The listing builds one solid part. Answer for the finished solid, in the listing's coordinates (mm). A direction names the side the tool comes from. Coordinates: 2 decimals unless noted, no trailing zeros. Loops run counter-clockwise (first coordinate to the right, second up) from the corner with the lowest first, then second, coordinate; pieces in that order, holes last. Notation, with made-up numbers: M 43,57.25 L 68,57.25 A23 ccw 68,83.25 Z; hole C 46.25,44.25 d4. An arc over 180 degrees is marked long. Return JSON: item names as keys, results as strings. Group by question number.
1. Section D-D (z = 17.5) is taken. Write down the section's boundary in (x, y).
2. Section C-C (z = -3.5) is taken. Write down the section's boundary in (x, y).
3. Which of the six approach directions +Z, -Z, +X, -X, +Y, -Y give full straight-line access (tool end or side, diameter ignored) to faces 5 (the face through (-24.6, 2, 0)), 6 (the face through (1.14, 1.48, -59.99))?
4. Section B-B (y = 1.5) is taken. Count the separate pieces of the cut face and the enclosed holes in it, then the cut area to 3 significant figures.
5. The mould has two halves that part along Z. Classify faces 1 (the face through (-1, 3, -1)), 2 (the face through (-41, 2, -12.9)), 3 (the face through (42, 2, -12.9)), 4 (the face through (-1.14, 1.48, 59.99)): pulls with the +Z half, pulls with the -Z half, needs draft (parallel to the pull), parting line crosses it, or undercut.
6. Given P1, Ø2, axis at x = -24.07, z = -45.64, coming from the -Y side; P2, Ø3, axis at x = -19, z = -14.5, coming from the -Y side; P3, Ø1.5, axis at y = 1.5, z = 0, coming from the -X side; P4, Ø1.4, axis at x = -27.5, y = 1, coming from the -Z side, each flat-ended and moving along its own axis, determine where each tip first touches the part or whether it passes through.
7. Section A-A (x = -30) is taken. Write down the section's boundary in (y, z).
8. Straight lines are drawn through the part: L1, parallel to Z at x = -25, y = 2.85; L2, parallel to Z at x = -39, y = 1.55; L3, parallel to Z at x = -0.5, y = 1.1. For each, find the intervals that lie inside material, in ascending order. Write a range as from..to.
```python
from build123d import *

# Parameters (mm, degrees)
SKETCH1_R           = 60
BOSS_EXTRUDE1_DEPTH = 3
SKETCH2_R           = 1.25
CUT_EXTRUDE1_DEPTH  = 4
CUT_EXTRUDE9_DEPTH  = 4
SKETCH5_R           = 0.9
BOSS_EXTRUDE2_DEPTH = 5
SKETCH7_R           = 0.9
BOSS_EXTRUDE3_DEPTH = 5
SKETCH8_R           = 0.9
BOSS_EXTRUDE4_DEPTH = 5
SKETCH9_R           = 0.9
BOSS_EXTRUDE5_DEPTH = 5


with BuildPart() as part:
    # Sketch1 → Boss-Extrude1 (new body)
    with BuildSketch(Plane(origin=(0, 0, 0), x_dir=(1, 0, 0), z_dir=(0, 1, 0))):
        Circle(SKETCH1_R)
    extrude(amount=BOSS_EXTRUDE1_DEPTH)

    # Sketch2 → Cut-Extrude1 (cut, through all)
    with BuildSketch(Plane(origin=(0, 3, 0), x_dir=(1, 0, 0), z_dir=(0, 1, 0))):
        with Locations((-42.393550358, 29.002085895)):
            Circle(SKETCH2_R)
        with Locations((42.606449642, 29.002085895)):
            Circle(SKETCH2_R)
        with Locations((42.606449642, -29.002085895)):
            Circle(SKETCH2_R)
        with Locations((-42.393550358, -29.002085895)):
            Circle(SKETCH2_R)
        with Locations((-24.073102507, 45.644631202)):
            Circle(SKETCH2_R)
        with Locations((24.073102507, 45.644631202)):
            Circle(SKETCH2_R)
        with Locations((24.073102507, -45.644631202)):
            Circle(SKETCH2_R)
        with Locations((-24.073102507, -45.644631202)):
            Circle(SKETCH2_R)
    extrude(amount=-CUT_EXTRUDE1_DEPTH, mode=Mode.SUBTRACT)

    # Sketch4 → Cut-Extrude9 (cut, through all)
    with BuildSketch(Plane(origin=(0, 3, 0), x_dir=(1, 0, 0), z_dir=(0, 1, 0))):
        with BuildLine():
            Line((-24.6, 12.9), (-58.596842918, 12.9))
            ThreePointArc((-58.596842918, 12.9), (-60, 0), (-58.596842918, -12.9))
            Line((-58.596842918, -12.9), (-24.6, -12.9))
            Line((-24.6, -12.9), (-24.6, 12.9))
        make_face()
        with BuildLine():
            Line((58.596842918, 12.9), (24.6, 12.9))
            Line((24.6, 12.9), (24.6, 0))
            Line((24.6, 0), (60, 0))
            ThreePointArc((60, 0), (59.648179248, 6.488043808), (58.596842918, 12.9))
        make_face()
        with BuildLine():
            Line((60, 0), (24.6, 0))
            Line((24.6, 0), (24.6, -12.9))
            Line((24.6, -12.9), (58.596842918, -12.9))
            ThreePointArc((58.596842918, -12.9), (59.648179248, -6.488043808), (60, 0))
        make_face()
    extrude(amount=-CUT_EXTRUDE9_DEPTH, mode=Mode.SUBTRACT)

    # Sketch5 → Boss-Extrude2 (add)
    with BuildSketch(Plane.XY.offset(-12.9)):
        with Locations((27.6, 1.5)):
            Circle(SKETCH5_R)
    extrude(amount=BOSS_EXTRUDE2_DEPTH)

    # Sketch7 → Boss-Extrude3 (add)
    with BuildSketch(Plane(origin=(0, 0, 12.9), x_dir=(-1, 0, 0), z_dir=(0, 0, -1))):
        with Locations((-27.6, 1.5)):
            Circle(SKETCH7_R)
    extrude(amount=BOSS_EXTRUDE3_DEPTH)

    # Sketch8 → Boss-Extrude4 (add)
    with BuildSketch(Plane.XY.offset(-12.9)):
        with Locations((-27.6, 1.5)):
            Circle(SKETCH8_R)
    extrude(amount=BOSS_EXTRUDE4_DEPTH)

    # Sketch9 → Boss-Extrude5 (add)
    with BuildSketch(Plane(origin=(0, 0, 12.9), x_dir=(-1, 0, 0), z_dir=(0, 0, -1))):
        with Locations((27.6, 1.5)):
            Circle(SKETCH9_R)
    extrude(amount=BOSS_EXTRUDE5_DEPTH)


solid = part.part
```
Worked out:
{
 "1": {"outline": "M -57.39,0 L 57.39,0 L 57.39,3 L -57.39,3 Z"},
 "2": {"outline": "M -24.6,0 L 24.6,0 L 24.6,3 L -24.6,3 Z"},
 "3": {"face 5": "+Y, -Y", "face 6": "-Z, +Y, -Y"},
 "4": {"separate pieces": "1", "enclosed holes": "8", "area": "9,500 mm^2"},
 "5": {"face 1": "needs draft", "face 2": "undercut", "face 3": "undercut", "face 4": "pulls with the +Z half"},
 "6": {"P1": "through", "P2": "y = 0", "P3": "x = -24.6", "P4": "z = -53.68"},
 "7": {"outline": "M 0,-51.96 L 3,-51.96 L 3,-12.9 L 0,-12.9 Z; M 0,12.9 L 3,12.9 L 3,51.96 L 0,51.96 Z"},
 "8": {"L1": "-54.54..-46.48, -44.81..-12.9, 12.9..44.81, 46.48..54.54", "L2": "-45.6..-12.9, 12.9..45.6", "L3": "-60..60"}
}
